Job drawing, mm, ordinate dimensions from the low corner. One solid piece. A direction names the side the tool comes from. Coordinates: 2 decimals unless noted, no trailing zeros. Order: outer loops, then holes, each group sorted by start corner. A loop starts at its lowest first (then second) coordinate and runs counter-clockwise, first axis right, second up. Notation, with made-up numbers: (54, 56.25) - (80, 56.25) arc R24 ccw to (80, 89.25) - close; hole circle Ø7 at (89.25, 21.5). An arc over 180 degrees is marked (long way). Write each question's results on one line, items separated by ' | '. Start each with the question number.
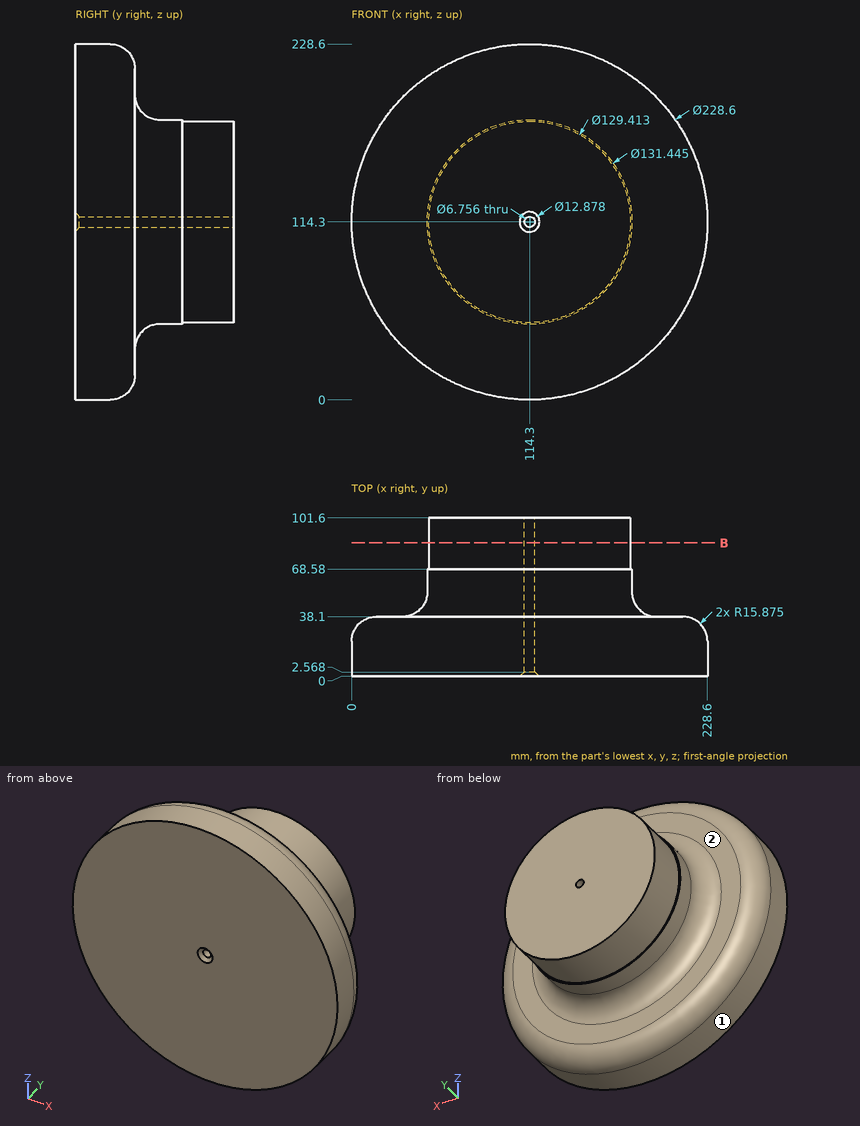
Item 1: Slice it at B-B (y = 85.5). Write the cut outline in (x, z).
Item 2: Probe probe 1 along X at (y, z) = (68, 114) (1 decimal); probe 2 along X at (y, z) = (71.5, 114.3); probe 3 along Y at (x, z) = (202, 133). List the from-to ranges inside material, lowest first.
Item 3: Flat gauge pins, fed straight in: P1, Ø12, axis at y = 68.5, z = 81, coming from the +X side (1 decimal); P2, Ø8, axis at x = 100, y = 76, coming from the +Z side; P3, Ø12, axis at x = 153.5, y = 26.5, coming from the +Z side; P4, Ø5, axis at y = 41.5, z = 23.5, coming from the +X side. Where does each tip first touch, or does it go through?
Item 4: Which spindle directions (+Z, -Z, +X, -X, +Y, -Y) get a long thin tool onto all of the face, cutting with end or side? Do the marked faces 1 and 2. Say none if no direction does.
Resolved:
1) outline: circle Ø129.41 at (114.3, 114.3); hole circle Ø6.76 at (114.3, 114.3)
2) probe 1: 48.6 to 110.9, 117.7 to 180 | probe 2: 49.59 to 110.92, 117.68 to 179.01 | probe 3: 0 to 38.1
3) P1: x = 174.1 | P2: z = 178.18 | P3: z = 223.4 | P4: through
4) face 1: +Y, -Y | face 2: +Y
